The model under review builds one solid part; all positions refer to its coordinate system, in mm. A direction names the side the tool comes from. Round coordinates to 2 decimals unless told otherwise and drop trailing zeros. Loops run counter-clockwise (first coordinate to the right, second up) from the corner with the lowest first, then second, coordinate; pieces in that order, holes last. Notation, with made-up numbers: M -30.75,80 L -0.75,80 A18 cw -0.75,109 Z; hole C -10.75,-3.5 d8. An arc over 180 degrees is marked long. Return JSON: item names as keys, results as strings. Group by question number.
Q1. Consider section A-A (x = -8). State the section outline as (y, z) points, and give its area (3 significant figures).
Q2. Consider section B-B (y = 1). State the section outline as (x, z) points.
Q3. To check wall thickness, follow line 1 along X through (y, z) = (1.25, 3.9); line 2 along Y through (x, z) = (-4, 16); line 3 along Z through (x, y) = (2.25, 5.75). State the ranges of each line that lie inside material, in increasing order.
Q4. Consider section D-D (x = 2.5). State the section outline as (y, z) points, and give its area (3 significant figures).
Q5. Draft analysis for pull direction Z (two halves, no side actions). For faces 1 (the face through (-7.504, 0.811, 5.474)), 2 (the face through (-4.25, 3.23, 8.59)), 3 (the face through (10.9, 1, 0)), 4 (the face through (0, 1, -6.4)), state which applies: pulls with the +Z half, pulls with the -Z half, needs draft (parallel to the pull), parting line crosses it, or undercut.
Q6. Clearance check with flat-ended pins moving along their axes: pin 1 Ø6.5 at (x, z) = (1, 5.5) entering from +Y; pin 2 Ø1 at (x, y) = (-2, 3.5) entering from -Z; pin 3 Ø1.5 at (y, z) = (3.5, 1) entering from -X. State where each tip first meets the part, or that it passes through.
Q7. Consider section C-C (z = 3.9). State the section outline as (x, y) points, and give its area (3 significant figures).
Q8. For faces 5 (the face through (0, 4.6, 9)), 6 (the face through (4.25, 3.17, 8.59)), 7 (the face through (0, 4.8, 4)), 8 (the face through (0, 1.8, 9)), list the 3-axis set-ups (+Z, -Z, +X, -X, +Y, -Y) from which the entire face can be reached by the end or side of a thin tool; tool diameter is ignored.
from build123d import *

# Parameters (mm, degrees)
SKETCH1_W           = 21.8
SKETCH1_H           = 12.8
BOSS_EXTRUDE1_DEPTH = 1.6
SKETCH2_R           = 1.65
CUT_EXTRUDE1_DEPTH  = 1.6
BOSS_EXTRUDE2_DEPTH = 7.4
BOSS_EXTRUDE3_DEPTH = 2
BOSS_EXTRUDE4_DEPTH = 10


with BuildPart() as part:
    # Sketch1 → Boss-Extrude1 (new body)
    with BuildSketch(Plane(origin=(0, 0, 0), x_dir=(1, 0, 0), z_dir=(0, 1, 0))):
        Rectangle(SKETCH1_W, SKETCH1_H)
    extrude(amount=BOSS_EXTRUDE1_DEPTH)

    # Sketch2 → Cut-Extrude1 (cut)
    with BuildSketch(Plane(origin=(0, 1.6, 0), x_dir=(1, 0, 0), z_dir=(0, 1, 0))):
        with Locations(Location((-8, -3.9, 0), (0, 0, 270))):
            Circle(SKETCH2_R)
        with Locations(Location((8, -3.9, 0), (0, 0, 270))):
            Circle(SKETCH2_R)
    extrude(amount=-CUT_EXTRUDE1_DEPTH, mode=Mode.SUBTRACT)

    # Sketch3 → Boss-Extrude2 (add)
    with BuildSketch(Plane.XY.offset(7.6)):
        with BuildLine():
            Line((-2.85, 4.8), (2.85, 4.8))
            ThreePointArc((2.85, 4.8), (4.45, 3.2), (2.85, 1.6))
            Line((2.85, 1.6), (-2.85, 1.6))
            ThreePointArc((-2.85, 1.6), (-4.45, 3.2), (-2.85, 4.8))
        make_face()
    extrude(amount=-BOSS_EXTRUDE2_DEPTH)

    # Sketch4 → Boss-Extrude3 (add)
    with BuildSketch(Plane.XY.offset(7.6)):
        with BuildLine():
            Line((-2.85, 1.8), (2.85, 1.8))
            ThreePointArc((2.85, 1.8), (4.25, 3.2), (2.85, 4.6))
            Line((2.85, 4.6), (-2.85, 4.6))
            ThreePointArc((-2.85, 4.6), (-4.25, 3.2), (-2.85, 1.8))
        make_face()
    extrude(amount=BOSS_EXTRUDE3_DEPTH)

    # Sketch5 → Boss-Extrude4 (add)
    with BuildSketch(Plane.XY.offset(9.6)):
        with BuildLine():
            Line((-2.85, -0.2), (2.85, -0.2))
            ThreePointArc((2.85, -0.2), (6.25, 3.2), (2.85, 6.6))
            Line((2.85, 6.6), (-2.85, 6.6))
            ThreePointArc((-2.85, 6.6), (-6.25, 3.2), (-2.85, -0.2))
        make_face()
    extrude(amount=BOSS_EXTRUDE4_DEPTH)


solid = part.part
Values:
{
 "1": {"outline": "M 0,-6.4 L 1.6,-6.4 L 1.6,2.25 L 0,2.25 Z; M 0,5.55 L 1.6,5.55 L 1.6,6.4 L 0,6.4 Z", "area": "15.2 mm2"},
 "2": {"outline": "M -10.9,-6.4 L 10.9,-6.4 L 10.9,6.4 L -10.9,6.4 Z; M -5.44,9.6 L 5.44,9.6 L 5.44,19.6 L -5.44,19.6 Z; hole C -8,3.9 d3.3; hole C 8,3.9 d3.3"},
 "3": {"line 1": "x = -10.9 to -9.65, -6.35 to 6.35, 9.65 to 10.9", "line 2": "y = 0 to 6.4", "line 3": "z = 9.6 to 19.6"},
 "4": {"outline": "M -0.2,9.6 L 1.8,9.6 L 1.8,7.6 L 1.6,7.6 L 1.6,6.4 L 0,6.4 L 0,-6.4 L 1.6,-6.4 L 1.6,0.2 L 4.8,0.2 L 4.8,7.6 L 4.6,7.6 L 4.6,9.6 L 6.6,9.6 L 6.6,19.6 L -0.2,19.6 Z", "area": "118 mm2"},
 "5": {"face 1": "undercut", "face 2": "undercut", "face 3": "needs draft", "face 4": "pulls with the -Z half"},
 "6": {"pin 1": "stops at y = 4.8", "pin 2": "stops at z = 0.2", "pin 3": "stops at x = -4.45"},
 "7": {"outline": "M -10.9,0 L -9.65,0 L -9.65,1.6 L -10.9,1.6 Z; M -6.35,0 L 6.35,0 L 6.35,1.6 L 2.85,1.6 A1.6 ccw 2.85,4.8 L -2.85,4.8 A1.6 ccw -2.85,1.6 L -6.35,1.6 Z; M 9.65,0 L 10.9,0 L 10.9,1.6 L 9.65,1.6 Z", "area": "50.6 mm2"},
 "8": {"face 5": "+X, -X, +Y", "face 6": "+X", "face 7": "-Z, +X, -X, +Y", "face 8": "+X, -X, -Y"}
}
